from build123d import *

# Parameters (mm, degrees)
BOSS_EXTRUDE1_DEPTH = 6.5
SKETCH2_W           = 4
SKETCH2_H           = 5
CUT_EXTRUDE1_DEPTH  = 7
CUT_EXTRUDE2_DEPTH  = 0.5
BOSS_EXTRUDE2_DEPTH = 10
SKETCH5_R           = 1.75
SKETCH5_R_2         = 0.5
CUT_EXTRUDE3_DEPTH  = 3.5
SKETCH7_R           = 1
CUT_EXTRUDE4_DEPTH  = 1


with BuildPart() as part:
    # Sketch1 → Boss-Extrude1 (new body)
    with BuildSketch(Plane(origin=(0, 0, 0), x_dir=(1, 0, 0), z_dir=(0, 1, 0))):
        Polygon((-4.748160816, 3.12599073), (-4.748160816, 3.933170407), (5.060522517, 3.933170407), (5.251839184, 3.933170407), (5.251839184, 2.992820323), (5.251839184, 1.607179677), (5.251839184, -2.13349626), (5.540514319, -1.966829593), (5.540514319, -2.966829593), (5.251839184, -2.800162927), (5.251839184, -3.666829593), (-4.748160816, -3.666829593), (-4.748160816, -2.800162927), (-4.459485681, -2.966829593), (-4.459485681, -1.966829593), (-4.748160816, -2.13349626), (-4.748160816, 1.740350084), align=None)
    extrude(amount=BOSS_EXTRUDE1_DEPTH)

    # Sketch2 → Cut-Extrude1 (cut)
    with BuildSketch(Plane(origin=(0, 0, -3.933170407), x_dir=(-1, 0, 0), z_dir=(0, 0, -1))):
        with Locations((-2.751839184, 3)):
            Rectangle(SKETCH2_W, SKETCH2_H)
        with Locations((2.248160816, 3)):
            Rectangle(SKETCH2_W, SKETCH2_H)
    extrude(amount=-CUT_EXTRUDE1_DEPTH, mode=Mode.SUBTRACT)

    # Sketch3 → Cut-Extrude2 (cut)
    with BuildSketch(Plane(origin=(0, 0, 0), x_dir=(-1, 0, 0), z_dir=(0, -1, 0))):
        with BuildLine():
            Line((-3.25, 3.933170407), (-2.25, 3.933170407))
            Line((-2.25, 3.933170407), (-2.25, -0.576829593))
            ThreePointArc((-2.25, -0.576829593), (-2.393517677, -0.923311916), (-2.74, -1.066829593))
            Line((-2.74, -1.066829593), (-2.76, -1.066829593))
            ThreePointArc((-2.76, -1.066829593), (-3.106482323, -0.923311916), (-3.25, -0.576829593))
            Line((-3.25, -0.576829593), (-3.25, 3.933170407))
        make_face()
        with BuildLine():
            Line((1.75, 3.933170407), (2.75, 3.933170407))
            Line((2.75, 3.933170407), (2.75, -0.576829593))
            ThreePointArc((2.75, -0.576829593), (2.606482323, -0.923311916), (2.26, -1.066829593))
            Line((2.26, -1.066829593), (2.24, -1.066829593))
            ThreePointArc((2.24, -1.066829593), (1.893517677, -0.923311916), (1.75, -0.576829593))
            Line((1.75, -0.576829593), (1.75, 3.933170407))
        make_face()
    extrude(amount=-CUT_EXTRUDE2_DEPTH, mode=Mode.SUBTRACT)

    # Sketch4 → Boss-Extrude2 (add)
    with BuildSketch(Plane(origin=(5.251839184, 0, 0), x_dir=(0, 0, -1), z_dir=(1, 0, 0))):
        Polygon((3.933170407, 6.5), (-3.666829593, 6.5), (-3.666829593, 7), (-2.066829593, 10), (2.933170407, 10), align=None)
    extrude(amount=-BOSS_EXTRUDE2_DEPTH)

    # Sketch5 → Cut-Extrude3 (cut)
    with BuildSketch(Plane(origin=(0, 10, 0), x_dir=(1, 0, 0), z_dir=(0, 1, 0))):
        with Locations(Location((-2.248160816, 0.433170407, 0), (0, 0, 270))):
            Circle(SKETCH5_R)
        with Locations(Location((2.751839184, 0.433170407, 0), (0, 0, 270))):
            Circle(SKETCH5_R)
        with Locations(Location((-2.248160816, -2.566829593, 0), (0, 0, 270))):
            Circle(SKETCH5_R_2)
        with Locations(Location((2.751839184, -2.566829593, 0), (0, 0, 270))):
            Circle(SKETCH5_R_2)
    extrude(amount=-CUT_EXTRUDE3_DEPTH, mode=Mode.SUBTRACT)

    # Sketch7 → Cut-Extrude4 (cut)
    with BuildSketch(Plane(origin=(0, 6.5, 0), x_dir=(1, 0, 0), z_dir=(0, 1, 0))):
        with Locations(Location((-2.25, 0.433170407, 0), (0, 0, 270))):
            Circle(SKETCH7_R)
        with Locations(Location((2.751839184, 0.433170407, 0), (0, 0, 270))):
            Circle(SKETCH7_R)
    extrude(amount=-CUT_EXTRUDE4_DEPTH, mode=Mode.SUBTRACT)


solid = part.part
Here's how the part is built. I have some questions about the finished solid (model axes, mm). A direction names the side the tool comes from. Coordinates: 2 decimals unless noted, no trailing zeros. Loops run counter-clockwise (first coordinate to the right, second up) from the corner with the lowest first, then second, coordinate; pieces in that order, holes last. Notation, with made-up numbers: (78.5, -26.5) -> (128.5, -26.5) arc R18 cw to (128.5, 5.5) -> close; hole circle Ø5 at (78, 24). An arc over 180 degrees is marked (long way). Use one line per item in the form item = value. Start each with the question number.
(1) If we section it at D-D (z = 0.25): Give the number of separate pieces and of enclosed holes in the cut face, then the cut area to 3 significant figures.
(2) If we section it at A-A (y = 2.75): Please give me the cut outline in (x, z), then the cut area to 3 significant figures.
(3) If we section it at C-C (x = 0): Please give me the cut outline in (y, z).
(4) Please list where these lines run through material, in increasing order: line 1 along X through (y, z) = (5, 1.5); line 2 along X through (y, z) = (4.5, 2.5); line 3 along Y through (x, z) = (1.25, 0).
(5) We'd pull the mould along X, two halves only. Please class faces 4 (the face through (0.752, 3, 0)), 5 (the face through (0, 3, -3.933)), 6 (the face through (5.541, 3.2, 2.5)): pulls with the +X half, pulls with the -X half, needs draft (parallel to the pull), parting line crosses it, or undercut.
(6) Will these pins go through, and if not, where does the flat tip stop? pin 1 (1.6 mm diameter, centred on x = 2.75, z = -0.43, fed in from +Y); pin 2 (1.2 mm diameter, centred on x = -2.5, y = 2, fed in from -Z); pin 3 (2.5 mm diameter, centred on x = -2.25, z = -0.43, fed in from +Y).
(7) On a 3-axis mill with a long thin cutter (end or side, diameter ignored), from which of +Z, -Z, +X, -X, +Y, -Y can I reach the whole of each face in a straight line? I mean faces 1 (the face through (2.774, 7.886, 2.067)), 2 (the face through (-2, 3, 3.067)), 3 (the face through (0.322, 8.479, 2.878)). Say none if no direction works.
(8) If we section it at B-B (y = 6): Please give me the cut outline in (x, z), then the cut area to 3 significant figures.
Verdict:
q1.separate_pieces = 3
q1.enclosed_holes = 0
q1.area = 33.5 mm²
q2.outline = (-4.75, -3.93) -> (-4.25, -3.93) -> (-4.25, 3.07) -> (-0.25, 3.07) -> (-0.25, -3.93) -> (0.75, -3.93) -> (0.75, 3.07) -> (4.75, 3.07) -> (4.75, -3.93) -> (5.25, -3.93) -> (5.25, 2.13) -> (5.54, 1.97) -> (5.54, 2.97) -> (5.25, 2.8) -> (5.25, 3.67) -> (-4.75, 3.67) -> (-4.75, 2.8) -> (-4.46, 2.97) -> (-4.46, 1.97) -> (-4.75, 2.13) -> close
q2.area = 20.0 mm²
q3.outline = (0, -3.93) -> (6.5, -3.93) -> (10, -2.93) -> (10, 2.07) -> (7, 3.67) -> (0, 3.67) -> close
q4.line_1 = -4.75 to -4.25, -0.25 to 0.75, 4.75 to 5.25
q4.line_2 = -4.46 to -4.25, -0.25 to 0.75, 4.75 to 5.54
q4.line_3 = 0 to 0.5, 5.5 to 6.5
q5.face_4 = undercut
q5.face_5 = needs draft
q5.face_6 = pulls with the +X half
q6.pin_1 = 0.5
q6.pin_2 = 3.07
q6.pin_3 = 6.5
q7.face_1 = +Y
q7.face_2 = -Z
q7.face_3 = +Z, +X, -X, +Y
q8.outline = (-4.75, -3.93) -> (5.25, -3.93) -> (5.25, 2.13) -> (5.54, 1.97) -> (5.54, 2.97) -> (5.25, 2.8) -> (5.25, 3.67) -> (-4.75, 3.67) -> (-4.75, 2.8) -> (-4.46, 2.97) -> (-4.46, 1.97) -> (-4.75, 2.13) -> close; hole circle Ø2 at (-2.25, -0.43); hole circle Ø2 at (2.75, -0.43)
q8.area = 69.7 mm²
